For this review, take the finished solid that the model builds, in its own axes (mm). A direction names the side the tool comes from. Give positions to 0.01 mm unless a question says otherwise; leave off trailing zeros. Write each loop counter-clockwise with the first axis right and the second up, starting at its lowest first coordinate (ties: lowest second). Pieces come first, ordered by that corner, then holes.
1) We need section C-C on y = 22.5. Give the boundary of the cut face in (x, z).
2) We need section B-B on x = -2.5. Give the boundary of the cut face in (y, z), and give its area (3 significant figures).
3) For P1, Ø1, axis at x = -1.5, y = 18.5, coming from the +Z side (3 decimals); P2, Ø6, axis at y = 24, z = -29, coming from the -X side; P3, Ø3, axis at x = 10.5, z = -62.5, coming from the -Y side; P4, Ø0.6, axis at x = 15, z = -58.5, coming from the -Y side, all flat-tipped, find the tip position at first contact; note any pin that passes through.
4) We need section A-A on z = -68.5. Give the boundary of the cut face in (x, y).
5) Machinability: for faces 4 (the face through (-6, -2, -51)), 5 (the face through (0, 14, -51)), 6 (the face through (14, 25, -49)), 7 (the face through (15, 24, -49)), which of the approach directions +Z, -Z, +X, -X, +Y, -Y give a long, thin tool a straight path to every point of the face, cutting with its end or side? Answer none if there is none.
6) Draft analysis for pull direction X (two halves, no side actions). For faces 1 (the face through (8, 28, -51)), 2 (the face through (9, 26, -49)), 3 (the face through (16, 26, -49)), state which applies: pulls with the +X half, pulls with the -X half, needs draft (parallel to the pull), parting line crosses it, or undercut.
7) Wall thickness on line 1 along Y through (x, z) = (-1.75, -7); line 2 along Y through (x, z) = (7, -73.5); line 3 along X through (y, z) = (19.5, -51): over which ranges is each line inside the solid? List them lowest first.
from build123d import *

# Parameters (mm, degrees)
SKETCH1_W            = 100
SKETCH1_H            = 26
BOSS_EXTRUDE1_DEPTH  = 2
BOSS_EXTRUDE2_DEPTH  = 100
MOVE_START           = -100
MOVE_FACE1_OUTLINE_W = 2
MOVE_FACE1_OUTLINE_H = 28
MOVE_FACE1_DEPTH     = 100
SKETCH5_W            = 100
SKETCH5_H            = 4
BOSS_EXTRUDE3_DEPTH  = 6
SKETCH6_W            = 100
SKETCH6_H            = 4
BOSS_EXTRUDE4_DEPTH  = 4


# Read off the part's stored shape, not the designer's step: Move Face1
with BuildPart() as part:
    # Sketch1 → Boss-Extrude1 (new body)
    with BuildSketch(Plane(origin=(0, 0, 0), x_dir=(0, 0, -1), z_dir=(1, 0, 0))):
        with Locations((50, 13)):
            Rectangle(SKETCH1_W, SKETCH1_H)
    extrude(amount=BOSS_EXTRUDE1_DEPTH)

    # Sketch2 → Boss-Extrude2 (add)
    with BuildSketch(Plane.XY):
        Polygon((2, 26), (2, 28), (-12, 28), (-12, 24), (-10, 24), (-10, 26), align=None)
    extrude(amount=-BOSS_EXTRUDE2_DEPTH)


with BuildPart() as body_2:
    # Mirror1: mirrored copy
    add(part.part.mirror(Plane.ZY.offset(-2)))

    # Move Face1 outline → Move Face1 (add)
    with BuildSketch(Plane.XY.offset(MOVE_START)):
        with Locations((1, 14)):
            Rectangle(MOVE_FACE1_OUTLINE_W, MOVE_FACE1_OUTLINE_H)
    extrude(amount=MOVE_FACE1_DEPTH)



with BuildPart() as body_2_2:
    # Sketch5 → Boss-Extrude3 (new body)
    with BuildSketch(Plane.ZY):
        with Locations((-50, -2)):
            Rectangle(SKETCH5_W, SKETCH5_H)
    extrude(amount=BOSS_EXTRUDE3_DEPTH)


with BuildPart() as body_2_1:
    add(body_2.part)

    add(body_2_2.part)  # Boss-Extrude4 merges body 2 2
    # Sketch6 → Boss-Extrude4 (add)
    with BuildSketch(Plane(origin=(0, 0, 0), x_dir=(0, 0, -1), z_dir=(1, 0, 0))):
        with Locations((50, -2)):
            Rectangle(SKETCH6_W, SKETCH6_H)
    extrude(amount=BOSS_EXTRUDE4_DEPTH)


solid = body_2_1.part
Results list:
1. outline: (0, -100) - (4, -100) - (4, 0) - (0, 0) - close
2. outline: (-4, -100) - (0, -100) - (0, 0) - (-4, 0) - close
2. area: 400 mm2
3. P1: passes through
3. P2: stops at x = 0
3. P3: stops at y = 26
3. P4: stops at y = 24
4. outline: (-6, -4) - (4, -4) - (4, 26) - (14, 26) - (14, 24) - (16, 24) - (16, 28) - (0, 28) - (0, 0) - (-6, 0) - close
5. face 4: +Z, -Z, -X, +Y, -Y
5. face 5: +Z, -Z, -X, +Y
5. face 6: +Z, -Z, -Y
5. face 7: +Z, -Z, +X, -Y
6. face 1: needs draft
6. face 2: undercut
6. face 3: pulls with the +X half
7. line 1: y = -4 to 0
7. line 2: y = 26 to 28
7. line 3: x = 0 to 4
